Build history of the part. All positions in model axes, mm. A direction names the side the tool comes from. Round coordinates to 2 decimals unless told otherwise and drop trailing zeros. Loops run counter-clockwise (first coordinate to the right, second up) from the corner with the lowest first, then second, coordinate; pieces in that order, holes last. Notation, with made-up numbers: M 1,82 L 15,82 A7 ccw 15,92 Z; hole C 81,3 d10. An arc over 180 degrees is marked long. Write each question's results on one line, items separated by ' | '. Start each with the question number.
```python
from build123d import *

# Parameters (mm, degrees)
SKETCH1_W           = 22.098
SKETCH1_H           = 22.098
BOSS_EXTRUDE1_DEPTH = 28.067
SKETCH2_W           = 25.7048
SKETCH2_H           = 25.7048
BOSS_EXTRUDE2_DEPTH = 25.7048
SKETCH3_W           = 22.098
SKETCH3_H           = 22.098
BOSS_EXTRUDE3_DEPTH = 28.067
FILLET1_R           = 1.27


with BuildPart() as part:
    # Sketch1 → Boss-Extrude1 (new body)
    with BuildSketch(Plane(origin=(0, 0, 0), x_dir=(1, 0, 0), z_dir=(0, 1, 0))):
        Rectangle(SKETCH1_W, SKETCH1_H)
    extrude(amount=BOSS_EXTRUDE1_DEPTH)

    # Sketch2 → Boss-Extrude2 (add)
    with BuildSketch(Plane(origin=(0, 28.067, 0), x_dir=(1, 0, 0), z_dir=(0, 1, 0))):
        Rectangle(SKETCH2_W, SKETCH2_H)
    extrude(amount=BOSS_EXTRUDE2_DEPTH)

    # Sketch3 → Boss-Extrude3 (add)
    with BuildSketch(Plane.XY.offset(12.8524)):
        with Locations((0, 40.9194)):
            Rectangle(SKETCH3_W, SKETCH3_H)
    extrude(amount=BOSS_EXTRUDE3_DEPTH)

    # Fillet1
    fillet1_edges = [part.edges().sort_by_distance(p)[0] for p in [
        (11.049, 29.8704, 26.8859),
        (11.049, 51.9684, 26.8859),
        (-11.049, 51.9684, 26.8859),
        (-11.049, 29.8704, 26.8859),
        (11.049, 14.0335, 11.049),
        (-11.049, 14.0335, 11.049),
        (-11.049, 14.0335, -11.049),
        (11.049, 14.0335, -11.049),
    ]]
    fillet(fillet1_edges, radius=FILLET1_R)


solid = part.part
```
Item 1: Tool access for faces 1 (the flat face through (11.049, 14, 0)), 2 (the flat face through (0, 51.968, 27)), 3 (the flat face through (-11.049, 14, 0)), 4 (the flat face through (0, 14, -11.049)), 5 (the cylindrical face through (-10.687, 51.586, 27.082)): list every direction of +Z, -Z, +X, -X, +Y, -Y with a clear straight run to the whole face (end or side of a thin tool).
Item 2: Saw through at C-C, the plane z = 33. Give the cut face in (x, y).
Item 3: Drop flat-ended pins along their axis: pin 1 (21.5 mm diameter, centred on y = 9.5, z = 3, fed in from +X); pin 2 (6 mm diameter, centred on x = -4.5, z = 27.5, fed in from +Y); pin 3 (6 mm diameter, centred on x = 3, z = 29.5, fed in from -Y). Give the stop position or say it passes through.
Item 4: Saw through at A-A, the plane y = 14. Give the cut face in (x, z), then the cut area to 3 significant figures.
Item 5: Saw through at B-B, the plane x = 2. Give the cut face in (y, z), then the cut area to 3 significant figures.
Item 6: Drill centre lines: line 1 along Z through (x, y) = (0.5, 16); line 2 along Z through (x, y) = (-11.25, 37.5). Where is each one in solid material? Low to high. Write a range as [from, to].
Working result:
1) face 1: +Z, -Z, +X, -Y | face 2: +Z, +X, -X, +Y | face 3: +Z, -Z, -X, -Y | face 4: -Z, +X, -X, -Y | face 5: +Z, -X, +Y
2) outline: M -11.05,31.14 A1.27 ccw -9.78,29.87 L 9.78,29.87 A1.27 ccw 11.05,31.14 L 11.05,50.7 A1.27 ccw 9.78,51.97 L -9.78,51.97 A1.27 ccw -11.05,50.7 Z
3) pin 1: stops at x = 11.05 | pin 2: stops at y = 51.97 | pin 3: stops at y = 29.87
4) outline: M -11.05,-9.78 A1.27 ccw -9.78,-11.05 L 9.78,-11.05 A1.27 ccw 11.05,-9.78 L 11.05,9.78 A1.27 ccw 9.78,11.05 L -9.78,11.05 A1.27 ccw -11.05,9.78 Z | area: 487 mm²
5) outline: M 0,-11.05 L 28.07,-11.05 L 28.07,-12.85 L 53.77,-12.85 L 53.77,12.85 L 51.97,12.85 L 51.97,40.92 L 29.87,40.92 L 29.87,12.85 L 28.07,12.85 L 28.07,11.05 L 0,11.05 Z | area: 1,900 mm²
6) line 1: z = [-11.05, 11.05] | line 2: z = [-12.85, 12.85]
